Read the model definition and answer for the solid it produces. Units are mm, in the model's axes. Face numbers are marked on the shaded views. A direction names the side the tool comes from. Round coordinates to 2 decimals unless told otherwise and drop trailing zeros. Write each loop counter-clockwise with the first axis right and the second up, starting at its lowest first coordinate (ties: lowest second). Pieces come first, ordered by that corner, then holes. Notation, with made-up numbers: (-24, 31.25) -> (26, 31.25) arc R27 cw to (26, 60.25) -> close; hole circle Ø11 at (-31, -14.75). An arc over 180 degrees is marked (long way). Return JSON: item names as keys, results as strings.
Autodesk Inventor part; units mm, degrees
ref_plane "Work Plane2" through (0, 0, 0) normal (0, 0, 1) x (1, 0, 0)
ref_plane "YZ Plane" through (0, 0, 0) normal (1, 0, 0) x (0, 1, 0)
ref_plane "XZ Plane" through (0, 0, 0) normal (0, 1, 0) x (-1, 0, 0)
ref_plane "Work Plane2" through (0, 0, 0) normal (0, 0, 1) x (1, 0, 0)
sketch "Sketch26" plane through (0, 0, 0) normal (0, 0, 1) x (1, 0, 0)
  circle A0 centre (0, 0) radius 60
  point P0 (0, 0)
extrude "Extrusion12" add sketch "Sketch26" along normal blind 15
sketch "Sketch28" plane through (0, 0, 0) normal (0, 0, -1) x (-1, 0, 0)
  circle A0 centre (0, 0) radius 30
  circle A1 centre (0, 0) radius 20 construction
  point P0 (0, 0)
  point P1 (20, 0)
  dimension "d225" = 40
hole "Hole13" at (-20, 0, 0) direction (0, 0, 1) diameter 6.6 end through all counterbore diameter 11 counterbore depth 6.8
pattern_circular "Circular Pattern10" count 6 over 360 about axis through (0, 0, 0) along (0, 0, 1) of "Hole13"
sketch "Sketch29" plane through (0, 0, 15) normal (0, 0, 1) x (1, 0, 0)
  circle A0 centre (-43.3013, 25) radius 2.4585
  circle A1 centre (-43.3013, -25) radius 2.4585
  point P0 (0, 0)
  point P1 (-43.0428, -24.2502)
  point P2 (-40.9021, -15.0744)
hole "Hole14" at (-43.3013, 25, 15) direction (0, 0, -1) diameter 6.6 depth 17.1 counterbore diameter 11 counterbore depth 6.8
pattern_circular "Circular Pattern11" count 6 over 360 about axis through (0, 0, 0) along (0, 0, 1) of "Hole14"
sketch "Sketch30" plane through (0, 0, 0) normal (0, 0, -1) x (-1, 0, 0)
  circle A0 centre (0, 35) radius 2.067 construction
  circle A1 centre (0, 35) radius 2.5
  point P0 (0, 0)
  dimension "d248" = 5
extrude "Extrusion13" cut sketch "Sketch30" against normal up to next
properties part number "base_connector" material "Copper"
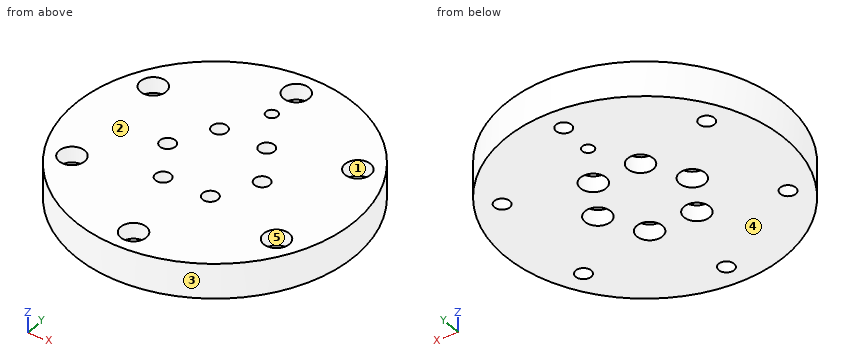
Item 1: Flat-ended cylindrical pins translate along their axes: pin 1 (2 mm diameter, centred on y = 9.5, z = 3, fed in from +X); pin 2 (1.5 mm diameter, centred on y = -18, z = 6, fed in from +X); pin 3 (3 mm diameter, centred on x = -42.5, z = 13, fed in from -Y). Find the tip coordinate at first contact, or state that the pin passes through.
Worked answers:
{"pin 1": "stops at x = 59.39", "pin 2": "stops at x = 57.47", "pin 3": "stops at y = -43.81"}
Item 2: A tool of negligible diameter and unlimited length cuts with its end or side. For the marked faces 4 and 5, from which of +Z, -Z, +X, -X, +Y, -Y can it reach the whole face along a straight path? Write none if from no direction.
Worked answers:
{"face 4": "-Z, +X, -X, +Y, -Y", "face 5": "+Z"}
Item 3: Section A-A (x = 0) is taken. Give the vertices of the cut face in (y, z).
Worked answers:
{"outline": "(-60, 0) -> (-53.3, 0) -> (-53.3, 8.2) -> (-55.5, 8.2) -> (-55.5, 15) -> (-60, 15) -> close; (-46.7, 0) -> (32.5, 0) -> (32.5, 15) -> (-44.5, 15) -> (-44.5, 8.2) -> (-46.7, 8.2) -> close; (37.5, 0) -> (46.7, 0) -> (46.7, 8.2) -> (44.5, 8.2) -> (44.5, 15) -> (37.5, 15) -> close; (53.3, 0) -> (60, 0) -> (60, 15) -> (55.5, 15) -> (55.5, 8.2) -> (53.3, 8.2) -> close"}
Item 4: Section D-D (y = 35) is taken. Give the vertices of the cut face in (x, z), then the cut area to 3 significant figures.
Worked answers:
{"outline": "(-48.73, 0) -> (-2.5, 0) -> (-2.5, 15) -> (-48.73, 15) -> close; (2.5, 0) -> (48.73, 0) -> (48.73, 15) -> (2.5, 15) -> close", "area": "1,390 mm2"}
Item 5: Section C-C (z = 1.75) is taken. State how many separate pieces and enclosed holes the cut face has, then the cut area to 3 significant figures.
Worked answers:
{"separate pieces": "1", "enclosed holes": "13", "area": "10,500 mm2"}
Item 6: Straight lines are drawn through the part: L1, parallel to Y at x = -40.5, z = 7.5; L2, parallel to X at y = 25, z = 3; L3, parallel to Y at x = -44.5, z = 2.5. For each, find the intervals that lie inside material, in ascending order. Write a range as [from, to].
Worked answers:
{"L1": "y = [-44.27, -26.74], [-23.26, 23.26], [26.74, 44.27]", "L2": "x = [-54.54, -46.6], [-40, 40], [46.6, 54.54]", "L3": "y = [-40.25, -28.07], [-21.93, 21.93], [28.07, 40.25]"}
Item 7: For a pull along Y with two mould halves and no side action, classify the marked faces 1, 2 and 3 as released by +Y, released by -Y, zero draft, split by the parting line, or undercut.
Worked answers:
{"face 1": "undercut", "face 2": "zero draft", "face 3": "split by the parting line"}
Item 8: Section B-B (y = 0) is taken. Give the vertices of the cut face in (x, z).
Worked answers:
{"outline": "(-60, 0) -> (-25.5, 0) -> (-25.5, 6.8) -> (-23.3, 6.8) -> (-23.3, 15) -> (-60, 15) -> close; (-16.7, 6.8) -> (-14.5, 6.8) -> (-14.5, 0) -> (14.5, 0) -> (14.5, 6.8) -> (16.7, 6.8) -> (16.7, 15) -> (-16.7, 15) -> close; (23.3, 6.8) -> (25.5, 6.8) -> (25.5, 0) -> (60, 0) -> (60, 15) -> (23.3, 15) -> close"}
